Autodesk Inventor part; units mm, degrees
ref_plane "Work Plane2" through (6.35, -3.175, -3.175) normal (0, -0.2586, -0.966) x (-0.5924, -0.7783, 0.2083)
ref_plane "YZ Plane" through (0, 0, 0) normal (1, 0, 0) x (0, 1, 0)
ref_plane "XZ Plane" through (0, 0, 0) normal (0, 1, 0) x (-1, 0, 0)
sketch "Sketch1" plane through (0, 0, 0) normal (0, 0, 1) x (1, 0, 0)
  line L0 (-6.35, -3.175) -> (6.35, -3.175) construction
  line L1 (6.35, -3.175) -> (6.35, 3.175)
  line L2 (6.35, 3.175) -> (-6.35, 3.175)
  line L3 (-6.35, 3.175) -> (-6.35, -3.175)
  line L4 (-6.35, -3.175) -> (6.35, 3.175) construction
  line L5 (6.35, -3.175) -> (-6.35, 3.175) construction
  line L6 (0, 6.0606) -> (0, -14.1385) construction
  line L7 (-6.35, -3.175) -> (-0.3234, -11.0927)
  line L8 (6.35, -3.175) -> (0.3234, -11.0927)
  arc A0 (-0.3234, -11.0927) -> (0.3234, -11.0927) centre (0, -10.8466) ccw
  point P0 (0, 0)
  dimension "d0" = 12.7
  dimension "d1" = 6.35
  dimension "d3" = 0.4064
extrude "Extrusion1" add sketch "Sketch1" along normal mid plane 6.35
sketch "Sketch2" plane through (0, 0, 0) normal (0, 0, 1) x (1, 0, 0)
  line L0 (6.35, -3.175) -> (6.35, 3.175)
  line L1 (-6.35, 3.175) -> (-6.35, -3.175)
  line L2 (-6.35, -3.175) -> (-0.3517, -13.5393)
  arc A0 (-0.3517, -13.5393) -> (0.3517, -13.5393) centre (0, -13.3358) ccw
  line L3 (6.35, -3.175) -> (0.3517, -13.5393)
  arc A1 (-0.3234, -11.0927) -> (0.3234, -11.0927) centre (0, -10.8466) ccw
  point P0 (0, 0)
  dimension "d9" = 0.4064
  dimension "d10" = 2.4892
sketch "Sketch3" plane through (-6.35, 3.175, 3.175) normal (0, 1, 0) x (1, 0, 0)
  line L0 (12.7, 0.9525) -> (11.5177, 2.9571)
  line L1 (11.5177, 3.3929) -> (12.7, 5.3975)
  line L2 (12.7, 5.3975) -> (12.7, 0.9525)
  arc A0 (11.5177, 3.3929) -> (11.5177, 2.9571) centre (11.8872, 3.175) ccw
  line L3 (12.7, 3.175) -> (11.8872, 3.175) construction
  point P0 (6.35, 3.175)
  dimension "d7" = 0.429
  dimension "d13" = 4.445
  dimension "d14" = 0.8128
sweep "Sweep1" cut profiles "Sketch3" path "Sketch2" path curves L0 L3 A0 L2 L1
ref_plane "Work Plane2" through (6.35, -3.175, -3.175) normal (0, -0.2586, -0.966) x (-0.5924, -0.7783, 0.2083)
ref_plane "Work Plane1" through (3.1636, -7.3612, -1.1019) normal (0, -0.2586, -0.966) x (-0.5924, -0.7783, 0.2083)
sketch "Sketch4" plane through (6.35, -3.175, -3.175) normal (0, -0.2586, -0.966) x (-0.5924, -0.7783, 0.2083)
  line L0 (10.1736, 0) -> (0, 0)
  line L1 (0, 0) -> (7.5232, 10.2319)
  line L2 (7.5232, 10.2319) -> (10.5567, 0.5211)
  ellipse E0 centre (10.1599, 0.4115) end of major axis (9.8209, 0.6607) minor radius 0.4064 (10.1736, 0) -> (10.5567, 0.5211) ccw
  point P0 (1.9521, 6.4464)
extrude "Extrusion2" cut sketch "Sketch4" along normal up to next
mirror "Mirror1" about plane through (0, 0, 0) normal (0, 0, 1) of "Extrusion2"
chamfer "Chamfer1" distance 0.2032 angle 45 4 edges at (6.35, 0, -3.175) (6.35, 0, 3.175) (-6.35, 0, -3.175) (-6.35, 0, 3.175)
sketch "Sketch5" plane through (5.5372, 3.175, 0) normal (0, 1, 0) x (1, 0, 0)
  circle A0 centre (-5.5372, 0) radius 2.3813
  dimension "d20" = 4.7625
extrude "Extrusion3" cut sketch "Sketch5" against normal blind 6.35
properties part number "Selector"
Input: part model. Units: mm. Frame: model coordinates. A direction names the side the tool comes from. Coordinates: 2 decimals unless noted, no trailing zeros. Write each loop counter-clockwise with the first axis right and the second up, starting at its lowest first coordinate (ties: lowest second). Pieces come first, ordered by that corner, then holes. Notation, with made-up numbers: M -13,39.25 L 11,39.25 A25 cw 11,69.25 Z; hole C 82,-33.5 d4. An arc over 180 degrees is marked long. Answer as a JSON object with one key per item and string values. Group by question number.
(1) Set-up query: faces 1 (the face through (5.767, 0.044, -1.234)), 2 (the face through (-4.29, -5.05, -0.79)), 3 (the face through (-5.751, -0.044, 1.206)). Return all of +Z, -Z, +X, -X, +Y, -Y with unobstructed straight access to the full face (end or side cutting, diameter ignored); none if empty.
(2) Section B-B on x = 0. Output: boundary loops of the cut face in (y, z) (3 decimals).
(3) Contact query for a flat-ended pin moving along its axis: P1, Ø3, axis at x = 3, y = -9.5, coming from the -Z side. Output: stop coordinate, or through.
(4) Mould query, pull axis Z, two halves, no side actions, for faces 4 (the face through (-0.674, -5.903, -2.445)), 5 (the face through (5.751, 0.044, 1.206)), 6 (the face through (3.128, -7.409, -1.402)). Classes: pulls with the +Z half, pulls with the -Z half, needs draft (parallel to the pull), parting line crosses it, or undercut.
(5) Ray query, line 1 along X through (y, z) = (-1.75, 0); line 2 along Z through (x, y) = (0, -1.5) (3 decimals); line 3 along X through (y, z) = (-2.75, -0.5). Return the intervals inside material, ascending. Write a range as [from, to].
Result set:
{
 "1": {"face 1": "+X, +Y, -Y", "face 2": "-X, -Y", "face 3": "-X, +Y, -Y"},
 "2": {"outline": "M -11.253,-1.013 L -3.175,-3.175 L 3.175,-3.175 L 3.175,-2.381 L -3.175,-2.381 L -3.175,2.381 L 3.175,2.381 L 3.175,3.175 L -3.175,3.175 L -11.253,1.013 Z"},
 "3": {"P1": "stops at z = -1.87"},
 "4": {"face 4": "pulls with the -Z half", "face 5": "undercut", "face 6": "needs draft"},
 "5": {"line 1": "x = [-5.11, -2.38], [2.38, 5.11]", "line 2": "z = [-3.175, -2.381], [2.381, 3.175]", "line 3": "x = [-5.33, -2.33], [2.33, 5.33]"}
}
